Verification items for the finished model (mm, model axes). Face numbers are marked on the shaded views. A direction names the side the tool comes from. Coordinates: 2 decimals unless noted, no trailing zeros. Order: outer loops, then holes, each group sorted by start corner. A loop starts at its lowest first (then second) coordinate and runs counter-clockwise, first axis right, second up. Notation, with made-up numbers: (30.5, -17) -> (78.5, -17) arc R13 cw to (78.5, -1) -> close; hole circle Ø10 at (85.5, 53.25). An arc over 180 degrees is marked (long way). Use CSV: the item, a comma, the result in double quotes. Start each with the question number.
1) Release check for a two-part mould opening along Y. For the marked faces 4, 5 and 6 record: released by +Y, released by -Y, zero draft, split by the parting line, or undercut.
2) Sectioned sample at D-D on x = 0.5. Record the boundary of the cut face in (y, z).
3) Scan lines: line 1 along Z through (x, y) = (23, 52.5); line 2 along X through (y, z) = (-7, 11); line 3 along Y through (x, z) = (-3, 23). Record each from-to range of solid material in increasing order.
4) Sectioned sample at A-A on y = 2.5. Record the boundary of the cut face in (x, z), then the cut area to 3 significant figures.
5) Tool access check on the marked faces 1, 2 and 3. Record the directions out of +Z, -Z, +X, -X, +Y, -Y that give a thin tool (end or side, any length) a straight path to the whole face; none if there is none.
6) Sectioned sample at C-C on z = 4.5. Give the number of separate pieces and of enclosed holes in the cut face, then the cut area to 3 significant figures.
7) Go/stop test with flat-tipped pins: pin 1 (10 mm diameter, centred on y = 31, z = 11, fed in from -X); pin 2 (10 mm diameter, centred on x = 22.5, y = 39, fed in from +Z); pin 3 (10 mm diameter, centred on y = 45.5, z = 23, fed in from +X). Record where each tip stops, or that it passes through.
8) Sectioned sample at B-B on z = 21. Record the boundary of the cut face in (x, y) (1 decimal).
from build123d import *

# Parameters (mm, degrees)
F0_R     = 14.2875
F1_DEPTH = 41.148
F0_R_2   = 6.35
F2_DEPTH = 11.176
F3_R     = 3.048
F5_DEPTH = 25.4
F7_DEPTH = 54.1640026378


with BuildPart() as f1:
    # F0 (on Top) → F1 (new body)
    with BuildSketch(Plane.XY):
        with BuildLine():
            ThreePointArc((-32.0825431228, 4.2204351945), (-14.1220308807, 11.6599229523), (-6.6825431228, 29.6204351945))
            ThreePointArc((-6.6825431228, 29.6204351945), (-14.1220308807, 47.5809474366), (-32.0825431228, 55.0204351945))
            ThreePointArc((-32.0825431228, 55.0204351945), (-57.4825431228, 29.6204351945), (-32.0825431228, 4.2204351945))
        make_face()
        with Locations((-32.0825431228, 29.6204351945)):
            Circle(F0_R, mode=Mode.SUBTRACT)
    extrude(amount=F1_DEPTH)

    # F0 (on Top) → F2 (join)
    with BuildSketch(Plane.XY):
        with BuildLine():
            ThreePointArc((-32.0825431228, 55.0204351945), (-14.1220308807, 47.5809474366), (-6.6825431228, 29.6204351945))
            ThreePointArc((-6.6825431228, 29.6204351945), (-14.1220308807, 11.6599229523), (-32.0825431228, 4.2204351945))
            Line((-32.0825431228, 4.2204351945), (8.057578387, -18.1441748871))
            ThreePointArc((8.057578387, -18.1441748871), (26.5875021064, -19.6841406643), (37.7656240054, -4.8255014786))
            Line((37.7656240054, -4.8255014786), (37.7656240054, 61.3704351945))
            ThreePointArc((37.7656240054, 61.3704351945), (27.6561701568, 78.1921216294), (8.057578387, 77.159943217))
            Line((8.057578387, 77.159943217), (-32.0825431228, 55.0204351945))
        make_face()
        with Locations((18.7174568772, -2.1295648055)):
            Circle(F0_R_2, mode=Mode.SUBTRACT)
        with Locations((18.7156240054, 61.3704351945)):
            Circle(F0_R_2, mode=Mode.SUBTRACT)
    extrude(amount=F2_DEPTH)

    # F3
    f3_edges = [f1.edges().sort_by_distance(p)[0] for p in [
        (-32.082543, 4.220435, 41.148),
    ]]
    fillet(f3_edges, radius=F3_R)

    # F4 (on face) → F5 (join)
    with BuildSketch(Plane.XY.offset(11.176)):
        with BuildLine():
            Line((34.4636240054, 26.4454351945), (34.4636240054, 32.7954351945))
            Line((34.4636240054, 32.7954351945), (-6.8817618849, 32.7954351945))
            ThreePointArc((-6.8817618849, 32.7954351945), (-6.6825431228, 29.6204351945), (-6.8817618849, 26.4454351945))
            Line((-6.8817618849, 26.4454351945), (34.4636240054, 26.4454351945))
        make_face()
    extrude(amount=F5_DEPTH)

    # F6 (on face) → F7 (cut, through all)
    with BuildSketch(Plane(origin=(0, 32.7954351945, 0), x_dir=(-1, 0, 0), z_dir=(0, 1, 0))):
        Polygon((-34.4636240054, 11.176), (6.8817618849, 36.576), (-34.4636240054, 36.576), align=None)
    extrude(amount=-F7_DEPTH, mode=Mode.SUBTRACT)


solid = f1.part
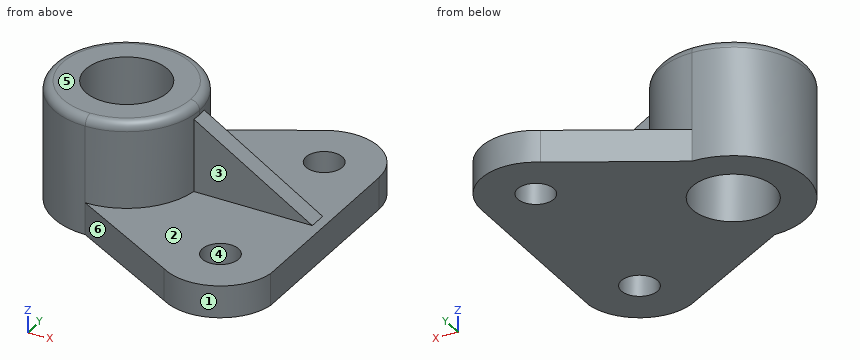
Answers follow:
1,face 4,"undercut"
1,face 5,"zero draft"
1,face 6,"released by -Y"
2,outline,"(-13.93, 0) -> (72.99, 0) -> (72.99, 11.18) -> (32.8, 11.18) -> (32.8, 32.04) -> (26.45, 32.04) -> (26.45, 11.18) -> (-13.93, 11.18) -> close"
3,line 1,"z = 0 to 11.18"
3,line 2,"x = -11.94 to 14.64, 22.79 to 37.33"
3,line 3,"y = 26.45 to 32.8"
4,outline,"(-28.99, 0) -> (14.37, 0) -> (14.37, 11.18) -> (-28.99, 11.18) -> close; (23.06, 0) -> (37.77, 0) -> (37.77, 11.18) -> (23.06, 11.18) -> close"
4,area,"649 mm²"
5,face 1,"+Z, -Z, -Y"
5,face 2,"+Z, +X"
5,face 3,"+Z, +X, -Y"
6,separate pieces,"1"
6,enclosed holes,"3"
6,area,"5,900 mm²"
7,pin 1,"stops at x = -57.48"
7,pin 2,"stops at z = 11.18"
7,pin 3,"stops at x = -9.13"
8,outline,"(-6.9, 26.4) -> (18.5, 26.4) -> (18.5, 32.8) -> (-6.9, 32.8) arc R25.4 ccw (long way) to start; hole circle Ø28.6 at (-32.1, 29.6)"
